Could you check a few things on this model? Use its own coordinates, in mm. Coordinates: 2 decimals unless noted, no trailing zeros. Order: outer loops, then holes, each group sorted by start corner. A loop starts at its lowest first (then second) coordinate and runs counter-clockwise, first axis right, second up. Notation, with made-up numbers: (69.25, -36.75) -> (83.25, -36.75) arc R10 cw to (83.25, -28.75) -> close; hole circle Ø7 at (30, -5). An arc over 180 degrees is marked (long way). Put each result on its own line as item: value. Start each with the question number.
Q1. Will these pins go through, and if not, where does the flat tip stop? pin 1 (2.5 mm diameter, centred on x = 33, y = 55, fed in from +Z); pin 2 (1.8 mm diameter, centred on x = 147, y = 55, fed in from +Z).
Q2. If we section it at C-C (z = 1.75): Please give me the cut outline in (x, y).
Q3. If we section it at A-A (y = 94): Please give me the cut outline in (x, z).
Q4. If we section it at B-B (x = 89): Please give me the cut outline in (y, z), and give its area (3 significant figures).
Q5. Please list where these lines run through material, in increasing order: line 1 along Y through (x, z) = (45, 2.3); line 2 along X through (y, z) = (99, 0.55); line 3 along Y through (x, z) = (52, 2.85).
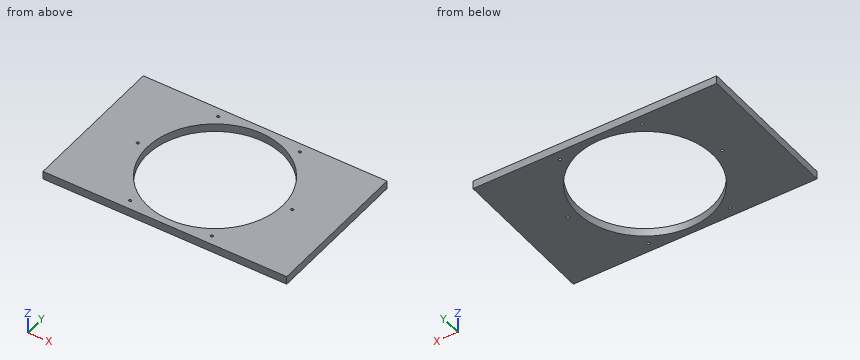
from build123d import *

# Parameters (mm, degrees)
SKETCH1_W           = 180
SKETCH1_H           = 110
BOSS_EXTRUDE1_DEPTH = 6
SKETCH2_R           = 50
CUT_EXTRUDE1_DEPTH  = 6
SKETCH4_R           = 1
CUT_EXTRUDE2_DEPTH  = 40


with BuildPart() as part:
    # Sketch1 → Boss-Extrude1 (new body)
    with BuildSketch(Plane.XY):
        with Locations((90, 55)):
            Rectangle(SKETCH1_W, SKETCH1_H)
    extrude(amount=BOSS_EXTRUDE1_DEPTH)

    # Sketch2 → Cut-Extrude1 (cut)
    with BuildSketch(Plane.XY):
        with Locations((90, 55)):
            Circle(SKETCH2_R)
    extrude(amount=CUT_EXTRUDE1_DEPTH, mode=Mode.SUBTRACT)

    # Sketch4 → Cut-Extrude2 (cut)
    with BuildSketch(Plane.XY):
        with Locations((59.794601939, 103.338741481)):
            Circle(SKETCH4_R)
        with Locations((120.205398061, 103.338741481)):
            Circle(SKETCH4_R)
        with Locations((147, 55)):
            Circle(SKETCH4_R)
        with Locations((120.205398061, 6.661258519)):
            Circle(SKETCH4_R)
        with Locations((59.794601939, 6.661258519)):
            Circle(SKETCH4_R)
        with Locations((33, 55)):
            Circle(SKETCH4_R)
    extrude(amount=CUT_EXTRUDE2_DEPTH, mode=Mode.SUBTRACT)


solid = part.part
The answers:
1. pin 1: z = 6
1. pin 2: through
2. outline: (0, 0) -> (180, 0) -> (180, 110) -> (0, 110) -> close; hole circle Ø2 at (33, 55); hole circle Ø100 at (90, 55); hole circle Ø2 at (59.79, 6.66); hole circle Ø2 at (59.79, 103.34); hole circle Ø2 at (120.21, 6.66); hole circle Ø2 at (120.21, 103.34); hole circle Ø2 at (147, 55)
3. outline: (0, 0) -> (58.71, 0) -> (58.71, 6) -> (0, 6) -> close; (121.29, 0) -> (180, 0) -> (180, 6) -> (121.29, 6) -> close
4. outline: (0, 0) -> (5.01, 0) -> (5.01, 6) -> (0, 6) -> close; (104.99, 0) -> (110, 0) -> (110, 6) -> (104.99, 6) -> close
4. area: 60.1 mm^2
5. line 1: 0 to 33.21, 76.79 to 110
5. line 2: 0 to 66.25, 113.75 to 180
5. line 3: 0 to 22.5, 87.5 to 110
